Autodesk Inventor part; units mm, degrees
ref_plane "YZ Plane" through (0, 0, 0) normal (1, 0, 0) x (0, 1, 0)
ref_plane "XZ Plane" through (0, 0, 0) normal (0, 1, 0) x (-1, 0, 0)
ref_plane "XY Plane" through (0, 0, 0) normal (0, 0, 1) x (1, 0, 0)
sketch "Boceto1" plane through (0, 0, 0) normal (1, 0, 0) x (0, 1, 0)
  line L0 (0, 0) -> (-16, 0)
  line L1 (-16, 0) -> (-16, -70)
  line L2 (0, -70) -> (0, 0)
  line L3 (0, -70) -> (0, -80)
  line L4 (0, -80) -> (-16, -80)
  line L5 (-16, -80) -> (-16, -70)
  dimension "d0" = 16
  dimension "d1" = 70
  dimension "d2" = 10
extrude "Extrusión1" add sketch "Boceto1" along normal blind 30
sketch "Boceto2" plane through (0, -16, -80) normal (0, 0, -1) x (-1, 0, 0)
  line L0 (0, 16) -> (-30, 16)
  line L1 (-15, 16) -> (-24, 16)
  line L2 (-24, 16) -> (-24, 0)
  line L3 (0, 0) -> (-30, 0)
  line L4 (-24, 0) -> (-30, 0)
  line L5 (-30, 16) -> (-30, 0)
  line L6 (-30, 0) -> (-30, 16)
  line L7 (-30, 16) -> (-24, 16)
  line L8 (-15, 16) -> (-6, 16)
  line L9 (-6, 16) -> (-6, 0)
  line L10 (0, 16) -> (0, 0)
  line L11 (-6, 0) -> (0, 0)
  line L12 (0, 0) -> (0, 16)
  line L13 (0, 16) -> (-6, 16)
  dimension "d5" = 9
  dimension "d6" = 9
extrude "Extrusión2" cut sketch "Boceto2" against normal blind 21 contours L10 L3 L9 L0 | L2 L3 L5 L0
sketch "Boceto3" plane through (24, -16, -80) normal (1, 0, 0) x (0, 0, -1)
  line L0 (-21, 16) -> (0, 16)
  line L1 (0, 16) -> (-8, 16)
  line L2 (-8, 16) -> (-8, 0)
  line L3 (0, 0) -> (-21, 0)
  arc A0 (-8, 0) -> (-8, 16) centre (-8, 8) ccw
  circle A1 centre (-8, 8) radius 3.5
  line L4 (0, 16) -> (0, 8)
  line L5 (0, 16) -> (0, 0)
  line L6 (0, 8) -> (0, 0)
  line L7 (0, 0) -> (-8, 0)
  point P0 (-80, 16)
  dimension "d9" = 8
  dimension "d10" = 7
extrude "Extrusión3" cut sketch "Boceto3" against normal blind 18 contours L0 L4 A0 | A1 L2 | L2 A1 | L5 L3 A0
properties part number "finger_long"
Geometry check sheet. Reference: the model listing, model coordinates, mm. A direction names the side the tool comes from. Round coordinates to 2 decimals unless told otherwise and drop trailing zeros. Loops run counter-clockwise (first coordinate to the right, second up) from the corner with the lowest first, then second, coordinate; pieces in that order, holes last. Notation, with made-up numbers: (-15, 70) -> (12, 70) arc R18 ccw to (12, 79) -> close; hole circle Ø10 at (74.5, 3). An arc over 180 degrees is marked (long way). Answer as a JSON object with one key per item and string values. Group by question number.
Item 1: Depth check by flat-ended pin: pin 1 Ø6.5 at (x, y) = (28, -5.5) entering from -Z; pin 2 Ø6 at (x, y) = (8.5, -4) entering from -Z; pin 3 Ø8 at (y, z) = (-8, -72) entering from +X. Enter the tip coordinate at first touch or a pass-through.
Item 2: Set-up check for faces 1 (the face through (6, -8, -67)), 2 (the face through (24, -8, -67)), 3 (the face through (15, -16, -37)): record each of +Z, -Z, +X, -X, +Y, -Y from which the full face is reachable in a straight line by a thin tool's end or side.
Item 3: Thickness scan on line 1 along Y through (x, z) = (14, -72); line 2 along Z through (x, y) = (17, -8); line 3 along Z through (x, y) = (5, -15). Record the ranges inside material, lowest first.
Item 4: Cross-section at D-D, the plane x = 3. Record the cut outline in (y, z).
Item 5: Cross-section at C-C, the plane y = -1.25. Record the cut outline in (x, z), plus the area to 3 significant figures.
Item 6: Cross-section at A-A, the plane y = -8. Record the cut outline in (x, z), plus the area to 3 significant figures.
Item 7: Cross-section at B-B, the plane z = -62. Record the cut outline in (x, y), plus the area to 3 significant figures.
Item 8: Release check for a two-part mould opening along Y. For faces 4 (the face through (15, 0, -37)), 5 (the face through (0, -8, -29)), 6 (the face through (15.126, -9.341, -75.233)), 7 (the face through (15, -8, -80)) record: pulls with the +Y half, pulls with the -Y half, needs draft (parallel to the pull), parting line crosses it, or undercut.
Determined:
{
 "1": {"pin 1": "stops at z = -59", "pin 2": "stops at z = -79.94", "pin 3": "stops at x = 24"},
 "2": {"face 1": "-Z, -X, +Y, -Y", "face 2": "-Z, +X, +Y, -Y", "face 3": "+Z, -Z, +X, -X, -Y"},
 "3": {"line 1": "y = -16 to -11.5, -4.5 to 0", "line 2": "z = -80 to -75.5, -68.5 to 0", "line 3": "z = -59 to 0"},
 "4": {"outline": "(-16, -59) -> (0, -59) -> (0, 0) -> (-16, 0) -> close"},
 "5": {"outline": "(0, -59) -> (6, -59) -> (6, -76.29) -> (24, -76.29) -> (24, -59) -> (30, -59) -> (30, 0) -> (0, 0) -> close", "area": "2,080 mm²"},
 "6": {"outline": "(0, -59) -> (6, -59) -> (6, -68.5) -> (24, -68.5) -> (24, -59) -> (30, -59) -> (30, 0) -> (0, 0) -> close; (6, -80) -> (24, -80) -> (24, -75.5) -> (6, -75.5) -> close", "area": "2,020 mm²"},
 "7": {"outline": "(6, -16) -> (24, -16) -> (24, 0) -> (6, 0) -> close", "area": "288 mm²"},
 "8": {"face 4": "pulls with the +Y half", "face 5": "needs draft", "face 6": "undercut", "face 7": "parting line crosses it"}
}
